The model under review builds one solid part; all positions refer to its coordinate system, in mm. Coordinates: 2 decimals unless noted, no trailing zeros. Loops run counter-clockwise (first coordinate to the right, second up) from the corner with the lowest first, then second, coordinate; pieces in that order, holes last. Notation, with made-up numbers: M 83,65 L 130,65 A9 cw 130,74 Z; hole C 30.5,60.5 d7. An arc over 180 degrees is marked long. Return JSON: item names as keys, results as strings.
```python
from build123d import *


# Not quite as in the source:
# - a fillet or chamfer that OpenCascade refuses, or shapes differently, is made with other operations: its cross-section is extruded or revolved along the edge and cut away or added


with BuildPart() as f1:
    # F0 (on Right) → F1 (revolve)
    with BuildSketch(Plane.YZ):
        Polygon((-59.2030874318, -23.7326024727), (54.3095125682, -23.7326024727), (54.3095125682, -6.2574024727), (50.3471125682, -6.2574024727), (50.3471125682, -17.3826024727), (-58.7138126601, -17.3826024727), align=None)
    revolve(axis=Axis((0, 27.4040363729, 0), (0, 1, 0)))

    # F2: fillet of radius 6.35 on 2 edges, made by hand

    # F2_s1 → F2_t2 (revolve, cut)
    with BuildSketch(Plane.YZ):
        with BuildLine():
            ThreePointArc((-52.3638126601, -23.7326024727), (-56.8539407206, -21.8727305333), (-58.7138126601, -17.3826024727))
            Line((-58.7138126601, -17.3826024727), (-58.8408126601, -17.3826024727))
            ThreePointArc((-58.8408126601, -17.3826024727), (-59.0850747245, -20.5478458962), (-59.3297121104, -23.7228458962))
            Line((-59.3297121104, -23.7228458962), (-59.2030874318, -23.8596024727))
            Line((-59.2030874318, -23.8596024727), (-52.3638126601, -23.8596024727))
            Line((-52.3638126601, -23.8596024727), (-52.3638126601, -23.7326024727))
        make_face()
    revolve(axis=Axis((0, -59.2030874318, 0), (0, 1, 0)), mode=Mode.SUBTRACT)

    # F2_s3 → F2_t4 (revolve, cut)
    with BuildSketch(Plane.YZ):
        with BuildLine():
            ThreePointArc((47.9595125682, -23.7326024727), (52.4496406287, -21.8727305333), (54.3095125682, -17.3826024727))
            Line((54.3095125682, -17.3826024727), (54.4365125682, -17.3826024727))
            Line((54.4365125682, -17.3826024727), (54.4365125682, -23.8596024727))
            Line((54.4365125682, -23.8596024727), (47.9595125682, -23.8596024727))
            Line((47.9595125682, -23.8596024727), (47.9595125682, -23.7326024727))
        make_face()
    revolve(axis=Axis((0, 54.3095125682, 0), (0, 1, 0)), mode=Mode.SUBTRACT)


solid = f1.part
```
1. Add section B-B on z = 0. Give the boundary of the cut face in (x, y).
Check values:
{"outline": "M -23.73,-52.36 A6.35 ccw -17.38,-58.71 L -17.38,50.35 L -6.26,50.35 L -6.26,54.31 L -17.38,54.31 A6.35 ccw -23.73,47.96 Z; M 6.26,50.35 L 17.38,50.35 L 17.38,-58.71 A6.35 ccw 23.73,-52.36 L 23.73,47.96 A6.35 ccw 17.38,54.31 L 6.26,54.31 Z"}
2. Insertion check: pin 1 Ø4 at (x, y) = (10.5, 24.5) entering from +Z; pin 2 Ø21 at (x, z) = (0, 0) entering from -Y; pin 3 Ø8 at (y, z) = (-23, -6.5) entering from +X; pin 4 Ø17.5 at (x, z) = (8, -8) entering from -Y. Each pin has a flat end and moves straight along its axis. Give the tip position at first contact, or say it passes through.
Check values:
{"pin 1": "z = 22.16", "pin 2": "y = 50.35", "pin 3": "x = 23.6", "pin 4": "y = -58.71"}
3. Add section C-C on y = 38. Give the boundary of the cut face in (x, z), plus the area to 3 significant figures.
Check values:
{"outline": "C 0,0 d47.47; hole C 0,0 d34.77", "area": "820 mm²"}
4. Add section A-A on x = 0. Give the boundary of the cut face in (y, z).
Check values:
{"outline": "M -58.71,-17.38 A6.35 ccw -52.36,-23.73 L 47.96,-23.73 A6.35 ccw 54.31,-17.38 L 54.31,-6.26 L 50.35,-6.26 L 50.35,-17.38 Z; M -58.71,17.38 L 50.35,17.38 L 50.35,6.26 L 54.31,6.26 L 54.31,17.38 A6.35 ccw 47.96,23.73 L -52.36,23.73 A6.35 ccw Z"}
5. The part is to be moulded in two halves that separate along X. For faces 1 (the face through (-7.129, -1.5, -22.637)), 2 (the face through (6.1, 52.3, 1.4)), 3 (the face through (7, 54.31, 0)), say which applies: released by +X, released by -X, zero draft, split by the parting line, or undercut.
Check values:
{"face 1": "split by the parting line", "face 2": "undercut", "face 3": "zero draft"}
6. To check wall thickness, follow line 1 (X direction, y = 20, z = 0); line 2 (Y direction, x = -8, z = 0.5). State the ranges of each line that lie inside material, in increasing order.
Check values:
{"line 1": "-23.73 to -17.38, 17.38 to 23.73", "line 2": "50.35 to 54.31"}
